Here's the drawing with two shaded views (mm, measured from the low corner). I have some questions. A direction names the side the tool comes from. Give positions to 0.01 mm unless a question says otherwise; leave off trailing zeros. Write each loop counter-clockwise with the first axis right and the second up, starting at its lowest first coordinate (ties: lowest second). Pieces come first, ordered by that corner, then holes.
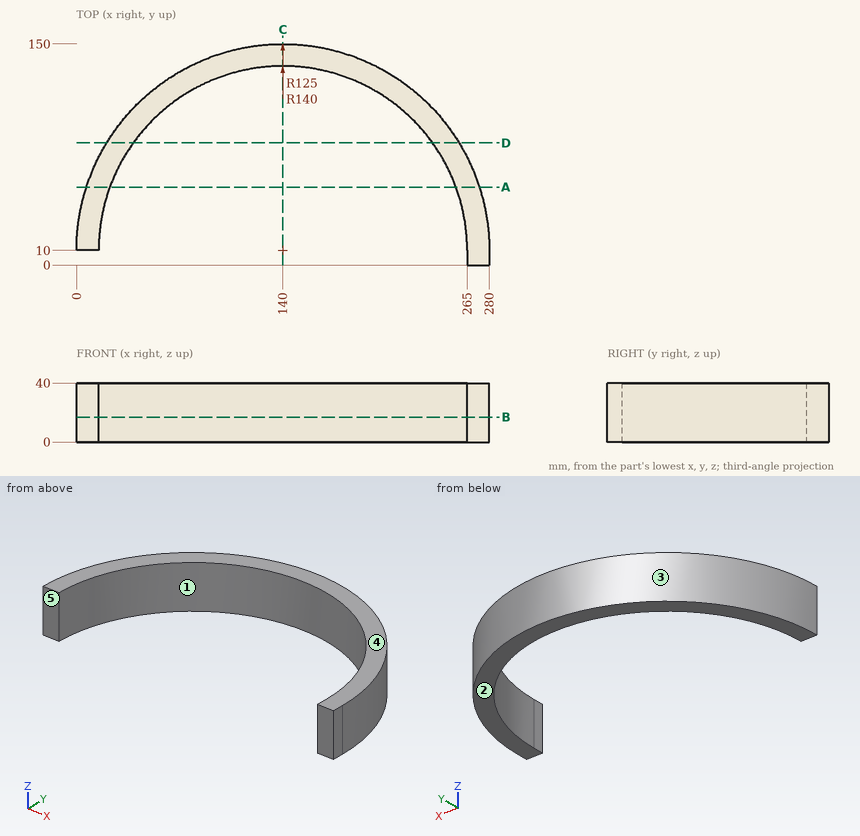
1) Suppose I cut it at C-C on x = 140. Write out the boundary of the cut face in (y, z).
Values follow:
outline: (135, 0) - (150, 0) - (150, 40) - (135, 40) - close
2) Suppose I cut it at D-D on y = 83. Write out the boundary of the cut face in (x, z).
Values follow:
outline: (20.54, 0) - (38.53, 0) - (38.53, 40) - (20.54, 40) - close; (241.47, 0) - (259.46, 0) - (259.46, 40) - (241.47, 40) - close
3) Suppose I cut it at B-B on z = 17. Write out the boundary of the cut face in (x, y), plus the area to 3 significant figures.
Values follow:
outline: (0, 10) - (15, 10) arc R125 cw to (265, 10) - (265, 0) - (280, 0) - (280, 10) arc R140 ccw to start
area: 6,390 mm2
4) If we mould it in two halves opening along X, with no side actions, what happens to the marked faces 1, 2 and 3? For each: +X half, -X half, draft (parallel to the pull), parting line (faces both ways), or undercut.
Values follow:
face 1: undercut
face 2: draft
face 3: parting line
5) For pin 1 Ø3 at (y, z) = (5, 17) entering from -X; pin 2 Ø1.5 at (x, z) = (251.5, 7) entering from +Y; pin 3 Ø2 at (x, z) = (223.5, 23) entering from -Y, each with a flat end and sliding along its axis, tell me the tip position at first contact or that it passes through.
Values follow:
pin 1: stops at x = 265
pin 2: stops at y = 95.64
pin 3: stops at y = 102.11
6) Please list where these lines run through material, in increasing order: L1, parallel to X at y = 85.5, z = 11.5; L2, parallel to X at y = 85, z = 23; L3, parallel to Y at x = 71.5, z = 28.
Values follow:
L1: x = 22.1 to 40.38, 239.62 to 257.9
L2: x = 21.78 to 40, 240 to 258.22
L3: y = 114.56 to 132.1
7) For the marked faces 4 and 5, which set-ups out of +Z, -Z, +X, -X, +Y, -Y let a thin tool reach every point of the face, with its end or its side?
Values follow:
face 4: +Z, +X, -X, +Y, -Y
face 5: +Z, -Z, -X, -Y
8) Suppose I cut it at A-A on y = 53. Write out the boundary of the cut face in (x, z), plus the area to 3 significant figures.
Values follow:
outline: (6.77, 0) - (22.63, 0) - (22.63, 40) - (6.77, 40) - close; (257.37, 0) - (273.23, 0) - (273.23, 40) - (257.37, 40) - close
area: 1,270 mm2
